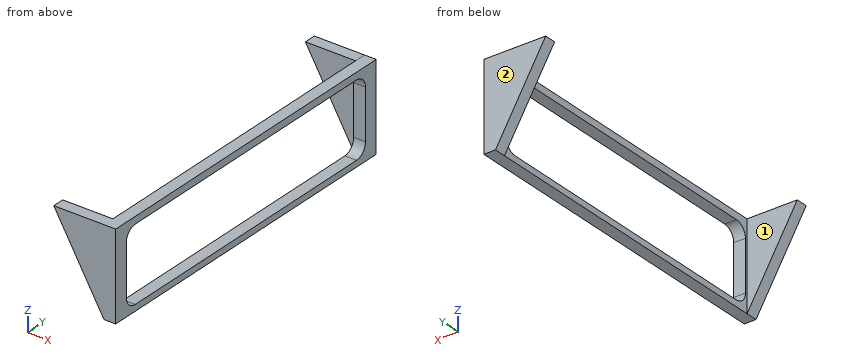
from build123d import *

# Parameters (mm, degrees)
F0_W     = 2.142924
F0_H     = 22.22561
F1_DEPTH = 3
F3_DEPTH = 3
F5_DEPTH = 3


with BuildPart() as f1:
    # F0 (on Right) → F1 (new body)
    with BuildSketch(Plane.YZ):
        Polygon((-41.607222, 6.203198), (-41.607222, -6.416802), (-41.607222, -11.112805), (41.562778, -11.112805), (41.562778, 11.112805), (-41.607222, 11.112805), align=None)
        with BuildLine():
            ThreePointArc((-40.136308, 6.302186), (-39.257629, 8.423506), (-37.136308, 9.302186))
            Line((-37.136308, 9.302186), (37.091864, 9.302186))
            ThreePointArc((37.091864, 9.302186), (39.213184, 8.423506), (40.091864, 6.302186))
            Line((40.091864, 6.302186), (40.091864, -6.51579))
            ThreePointArc((40.091864, -6.51579), (39.213184, -8.63711), (37.091864, -9.51579))
            Line((37.091864, -9.51579), (-37.136308, -9.51579))
            ThreePointArc((-37.136308, -9.51579), (-39.257629, -8.63711), (-40.136308, -6.51579))
            Line((-40.136308, -6.51579), (-40.136308, 6.302186))
        make_face(mode=Mode.SUBTRACT)
        Polygon((-41.607222, -11.112805), (-41.607222, -6.416802), (-41.607222, 6.203198), (-41.607222, 11.112805), (-43.705702, 11.112805), (-43.705702, -11.112805), align=None)
        with Locations((42.63424, 0)):
            Rectangle(F0_W, F0_H)
    extrude(amount=F1_DEPTH)

    # F2 (on face) → F3 (join)
    with BuildSketch(Plane.XZ.offset(43.705702)):
        Polygon((0, -11.112805), (0, 11.112805), (-12.831961, 11.112805), align=None)
    extrude(amount=-F3_DEPTH)

    # F4 (on face) → F5 (join)
    with BuildSketch(Plane(origin=(0, 43.705702, 0), x_dir=(-1, 0, 0), z_dir=(0, 1, 0))):
        Polygon((12.824409, 11.117161), (0, 11.112805), (0, -11.112805), align=None)
    extrude(amount=-F5_DEPTH)


solid = f1.part
Input: part model. Units: mm. Frame: model coordinates. Face numbers are marked on the shaded views. A direction names the side the tool comes from. Coordinates: 2 decimals unless noted, no trailing zeros. Loops run counter-clockwise (first coordinate to the right, second up) from the corner with the lowest first, then second, coordinate; pieces in that order, holes last. Notation, with made-up numbers: (-15, 22.5) -> (32, 22.5) arc R14 ccw to (32, 37.5) -> close; hole circle Ø9 at (35, 58.25). An arc over 180 degrees is marked (long way). One line per item, written item: value.
(1) Cut plane D-D (x = -7). Output: boundary loops of the cut face in (y, z), then the cut area to 3 significant figures.
Answer below:
outline: (-43.71, 1.01) -> (-40.71, 1.01) -> (-40.71, 11.11) -> (-43.71, 11.11) -> close; (40.71, 1.02) -> (43.71, 1.02) -> (43.71, 11.12) -> (40.71, 11.12) -> close
area: 60.6 mm2
(2) Ray query, line 1 along Y through (x, z) = (2.75, -4.25); line 2 along Y through (x, z) = (-1.5, 5); line 3 along Z through (x, y) = (1.5, 31.5). Return the intervals inside material, ascending.
Answer below:
line 1: y = -43.71 to -40.14, 40.09 to 43.71
line 2: y = -43.71 to -40.71, 40.71 to 43.71
line 3: z = -11.11 to -9.52, 9.3 to 11.11
(3) Cut plane B-B (y = 18.5). Output: boundary loops of the cut face in (x, z).
Answer below:
outline: (0, -11.11) -> (3, -11.11) -> (3, -9.52) -> (0, -9.52) -> close; (0, 9.3) -> (3, 9.3) -> (3, 11.11) -> (0, 11.11) -> close
(4) Set-up query: the marked faces 1 and 2. Return all of +Z, -Z, +X, -X, +Y, -Y with unobstructed straight access to the full face (end or side cutting, diameter ignored); none if empty.
Answer below:
face 1: +Z, -Z, -X
face 2: +Z, -Z, +X, -X, +Y
(5) Pin query (flat end, axial travel): pin 1 Ø8 at (x, y) = (-6.5, 7) entering from +Z; pin 2 Ø2 at (x, y) = (1.5, 5) entering from +Z. Return the tip coordinate at first contact, or that it passes through.
Answer below:
pin 1: passes through
pin 2: stops at z = 11.11
(6) Cut plane C-C (z = 4.5). Output: boundary loops of the cut face in (x, y).
Answer below:
outline: (-9.01, -43.71) -> (3, -43.71) -> (3, -40.14) -> (0, -40.14) -> (0, -40.71) -> (-9.01, -40.71) -> close; (-9.01, 40.71) -> (0, 40.71) -> (0, 40.09) -> (3, 40.09) -> (3, 43.71) -> (-9.01, 43.71) -> close
(7) Cut plane A-A (x = 1). Output: boundary loops of the cut face in (y, z).
Answer below:
outline: (-43.71, -11.11) -> (43.71, -11.11) -> (43.71, 11.11) -> (-43.71, 11.11) -> close; hole (-40.14, -6.52) arc R3 ccw to (-37.14, -9.52) -> (37.09, -9.52) arc R3 ccw to (40.09, -6.52) -> (40.09, 6.3) arc R3 ccw to (37.09, 9.3) -> (-37.14, 9.3) arc R3 ccw to (-40.14, 6.3) -> close
